Geometry check sheet. Reference: the model listing, model coordinates, mm. Face numbers are marked on the shaded views. Coordinates: 2 decimals unless noted, no trailing zeros. Write each loop counter-clockwise with the first axis right and the second up, starting at its lowest first coordinate (ties: lowest second). Pieces come first, ordered by that corner, then holes. Notation, with made-up numbers: (-10.75, -38) -> (26.25, -38) arc R24 cw to (26.25, -27) -> close; hole circle Ø9 at (33, -23.5). An arc over 180 degrees is marked (long way). Use a Markdown table: item, result.
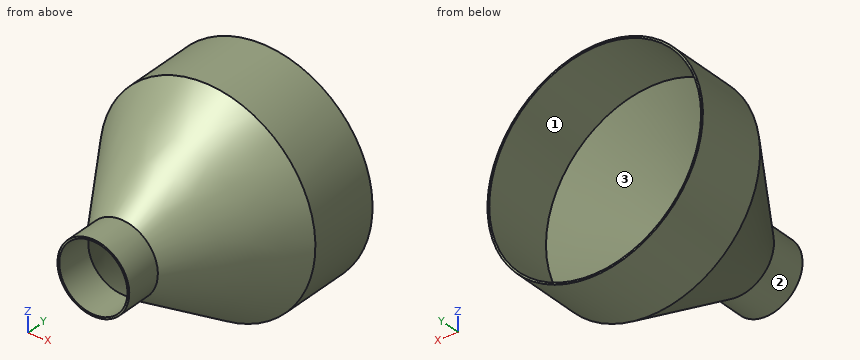
```python
from build123d import *

# Parameters (mm, degrees)
SKETCH1_W   = 40
SKETCH1_H   = 120
SKETCH1_H_2 = 80
SKETCH1_W_2 = 80
SKETCH1_H_3 = 40
SHELL2_T    = -2


with BuildPart() as part:
    # Sketch1 → Revolve3 (revolve)
    with BuildSketch(Plane.XY, mode=Mode.PRIVATE) as revolve3_sk:
        with Locations((-20, 100)):
            Rectangle(SKETCH1_W, SKETCH1_H)
        with Locations((-20, 200)):
            Rectangle(SKETCH1_W, SKETCH1_H_2)
        with Locations((-80, 200)):
            Rectangle(SKETCH1_W_2, SKETCH1_H_2)
        Polygon((-40, 160), (-120, 160), (-40, 40), align=None)
        with Locations((-20, 20)):
            Rectangle(SKETCH1_W, SKETCH1_H_3)
    revolve(revolve3_sk.sketch.rotate(Axis((0, 249.803796798, 0), (0, -1, 0)), 270), axis=Axis((0, 249.803796798, 0), (0, -1, 0)))

    # Shell2
    shell2_openings = [part.faces().sort_by_distance(p)[0] for p in [
        (0, 240, 0),
        (0, 0, 0),
    ]]
    offset(amount=SHELL2_T, openings=shell2_openings, kind=Kind.INTERSECTION)


solid = part.part
```
Item 1: Section check D-D on y = 95.5. Record the boundary of the cut face in (x, z), then the cut area to 3 significant figures.
Answer block:
| item | result |
|---|---|
| outline | circle Ø154 at (0, 0); hole circle Ø149.19 at (0, 0) |
| area | 1,140 mm^2 |
Item 2: Section check C-C on y = 199. Record the boundary of the cut face in (x, z), then the cut area to 3 significant figures.
Answer block:
| item | result |
|---|---|
| outline | circle Ø240 at (0, 0); hole circle Ø236 at (0, 0) |
| area | 1,500 mm^2 |
Item 3: Depth check by flat-ended pin: P1, Ø3, axis at y = 100, z = -44, coming from the -X side; P2, Ø1, axis at y = 77, z = -28.5, coming from the -X side; P3, Ø2, axis at x = -70.5, z = -36, coming from the +Y side (3 decimals). Enter the tip coordinate at first touch or a pass-through.
Answer block:
| item | result |
|---|---|
| P1 | stops at x = -68.35 |
| P2 | stops at x = -58.49 |
| P3 | stops at y = 103.845 |
Item 4: Thickness scan on L1, parallel to X at y = 10, z = 0; L2, parallel to X at y = 185, z = 0; L3, parallel to Z at x = -9, y = 30.5. Record the ranges inside material, lowest first. Write a range as [from, to].
Answer block:
| item | result |
|---|---|
| L1 | x = [-40, -38], [38, 40] |
| L2 | x = [-120, -118], [118, 120] |
| L3 | z = [-38.97, -36.92], [36.92, 38.97] |
Item 5: Mould release check, pull along Z, two halves, no side actions. Record for the marked faces 1, 2 and 3: +Z half, -Z half, draft (parallel to the pull), parting line (faces both ways), or undercut.
Answer block:
| item | result |
|---|---|
| face 1 | undercut |
| face 2 | parting line |
| face 3 | undercut |
Item 6: Section check B-B on x = 0. Record the boundary of the cut face in (y, z), then the cut area to 3 significant figures.
Answer block:
| item | result |
|---|---|
| outline | (0, -40) -> (40, -40) -> (160, -120) -> (240, -120) -> (240, -118) -> (160.61, -118) -> (40.61, -38) -> (0, -38) -> close; (0, 38) -> (40.61, 38) -> (160.61, 118) -> (240, 118) -> (240, 120) -> (160, 120) -> (40, 40) -> (0, 40) -> close |
| area | 1,060 mm^2 |
Item 7: Section check A-A on z = 0. Record the boundary of the cut face in (x, y), then the cut area to 3 significant figures.
Answer block:
| item | result |
|---|---|
| outline | (-120, 160) -> (-40, 40) -> (-40, 0) -> (-38, 0) -> (-38, 40.61) -> (-118, 160.61) -> (-118, 240) -> (-120, 240) -> close; (38, 0) -> (40, 0) -> (40, 40) -> (120, 160) -> (120, 240) -> (118, 240) -> (118, 160.61) -> (38, 40.61) -> close |
| area | 1,060 mm^2 |
